from build123d import *

# Parameters (mm, degrees)
SKETCH1_W           = 228.6
SKETCH1_H           = 406.4
SKETCH1_R           = 14.2875
SKETCH1_R_2         = 4.7625
SKETCH1_W_2         = 136.525
SKETCH1_H_2         = 444.5
BOSS_EXTRUDE1_DEPTH = 63.5
SKETCH2_W           = 38.1
SKETCH2_H           = 495.3
CUT_EXTRUDE1_DEPTH  = 36.5125
SKETCH3_R           = 4.7625
CUT_EXTRUDE2_DEPTH  = 690.786561191
FILLET1_R           = 46.0375
CHAMFER1_SIZE       = 31.75


with BuildPart() as part:
    # Sketch1 → Boss-Extrude1 (new body)
    # profile 1 of 2: a face of its own
    with BuildSketch(Plane.XY):
        Rectangle(SKETCH1_W, SKETCH1_H)
        with Locations((0, -25.4)):
            Circle(SKETCH1_R, mode=Mode.SUBTRACT)
        with Locations((-50.174093823, -25.4)):
            Circle(SKETCH1_R_2, mode=Mode.SUBTRACT)
        with Locations((50.174093823, -25.4)):
            Circle(SKETCH1_R_2, mode=Mode.SUBTRACT)
    # profile 2 of 2: a face of its own
    with BuildSketch(Plane.XY):
        with Locations((0, -425.45)):
            Rectangle(SKETCH1_W_2, SKETCH1_H_2)
    extrude(amount=BOSS_EXTRUDE1_DEPTH)

    # Sketch2 → Cut-Extrude1 (cut)
    with BuildSketch(Plane(origin=(0, 0, 0), x_dir=(-1, 0, 0), z_dir=(0, 0, -1))):
        with Locations((0, -376.2375)):
            Rectangle(SKETCH2_W, SKETCH2_H)
    extrude(amount=-CUT_EXTRUDE1_DEPTH, mode=Mode.SUBTRACT)

    # Sketch3 → Cut-Extrude2 (cut, through all)
    with BuildSketch(Plane.ZY.offset(114.3)):
        with Locations(Location((19.05, -150.8125, 0), (0, 0, 270))):
            Circle(SKETCH3_R)
    extrude(amount=-CUT_EXTRUDE2_DEPTH, mode=Mode.SUBTRACT)

    # Fillet1
    fillet1_edges = [part.edges().sort_by_distance(p)[0] for p in [
        (68.2625, -203.2, 31.75),
        (-68.2625, -203.2, 31.75),
    ]]
    fillet(fillet1_edges, radius=FILLET1_R - 0.0001)  # a hair under: the kernel refuses the full size

    # Chamfer1
    chamfer1_edges = [part.edges().sort_by_distance(p)[0] for p in [
        (0, 203.2, 63.5),
    ]]
    chamfer(chamfer1_edges, length=CHAMFER1_SIZE)


solid = part.part
For this review, take the finished solid that the model builds, in its own axes (mm). A direction names the side the tool comes from. Coordinates: 2 decimals unless noted, no trailing zeros. Write each loop counter-clockwise with the first axis right and the second up, starting at its lowest first coordinate (ties: lowest second). Pieces come first, ordered by that corner, then holes. Notation, with made-up numbers: (27.5, 42) -> (83.5, 42) arc R19 cw to (83.5, 56) -> close; hole circle Ø3 at (-6.5, 62.25). An arc over 180 degrees is marked (long way). Write each question's results on one line, items separated by ' | '. Start each with the question number.
1) The part is to be moulded in two halves that separate along X. For faces 4 (the face through (68.262, -451, 31)), 5 (the face through (0, -128.588, 18)), 6 (the face through (-114.3, -3, 31)), say which applies: +X half, -X half, draft (parallel to the pull), parting line (faces both ways), or undercut.
2) Consider section C-C (y = -568.5). Write out the cut boundary in (x, z), plus the area to 3 significant figures.
3) Insertion check: pin 1 (3 mm diameter, centred on y = -413, z = 8.5, fed in from +X). The pin has a flat end and moves straight along its axis. Give the tip position at first contact, or say it passes through.
4) Consider section B-B (x = 0). Write out the cut boundary in (y, z).
5) For faces 1 (the face through (-2, -122, 0)), 2 (the face through (-19.05, -380, 18)), 3 (the face through (-68.262, -451, 31)), list the 3-axis set-ups (+Z, -Z, +X, -X, +Y, -Y) from which the entire face can be reached by the end or side of a thin tool; tool diameter is ignored.
6) Wall thickness on L1, parallel to X at y = -25, z = 34; L2, parallel to Y at x = -36.5, z = 20; L3, parallel to X at y = -370, z = 13.5: over which ranges is each line inside the solid? List them lowest first. Write a range as [from, to].
7) Consider section A-A (z = 54.5). Give the number of separate pieces and of enclosed holes in the cut face, plus the area to 3 significant figures.
Geometry says:
1) face 4: +X half | face 5: undercut | face 6: -X half
2) outline: (-68.26, 0) -> (-19.05, 0) -> (-19.05, 36.51) -> (19.05, 36.51) -> (19.05, 0) -> (68.26, 0) -> (68.26, 63.5) -> (-68.26, 63.5) -> close | area: 7,280 mm^2
3) pin 1: x = 68.26
4) outline: (-647.7, 0) -> (-623.89, 0) -> (-623.89, 36.51) -> (-128.59, 36.51) -> (-128.59, 0) -> (-39.69, 0) -> (-39.69, 63.5) -> (-647.7, 63.5) -> close; (-11.11, 0) -> (203.2, 0) -> (203.2, 31.75) -> (171.45, 63.5) -> (-11.11, 63.5) -> close
5) face 1: -Z, +X, -X, +Y, -Y | face 2: -Z | face 3: +Z, -Z, -X, -Y
6) L1: [-114.3, -54.92], [-45.43, -14.28], [14.28, 45.43], [54.92, 114.3] | L2: [-647.7, -155.48], [-146.15, 203.2] | L3: [-68.26, -19.05], [19.05, 68.26]
7) separate pieces: 1 | enclosed holes: 3 | area: 149,000 mm^2
